from build123d import *

# Parameters (mm, degrees)
SKETCH1_W                                      = 83.2
SKETCH1_H                                      = 74.2
BOSS_EXTRUDE1_DEPTH                            = 8
SHELL1_T                                       = -2
SKETCH2_R                                      = 4.5
SKETCH2_R_2                                    = 2.5
BOSS_EXTRUDE2_DEPTH                            = 4.6
SKETCH3_W                                      = 81.2
SKETCH3_H                                      = 72.2
CUT_EXTRUDE1_DEPTH                             = 1
SKETCH4_R                                      = 2.5
BOSS_EXTRUDE3_DEPTH                            = 0.5
CSK_FOR_M3_FLAT_HEAD_MACHINE_SCREW1_AT_2_COUNT = 2
CSK_FOR_M3_FLAT_HEAD_MACHINE_SCREW1_AT_2_PITCH = 45.11064176
CSK_FOR_M3_FLAT_HEAD_MACHINE_SCREW1_AT_3_COUNT = 2
CSK_FOR_M3_FLAT_HEAD_MACHINE_SCREW1_AT_3_PITCH = 45.11064176
CSK_FOR_M3_FLAT_HEAD_MACHINE_SCREW1_AT_4_COUNT = 2
CSK_FOR_M3_FLAT_HEAD_MACHINE_SCREW1_AT_4_PITCH = 58.2
FILLET1_R                                      = 2


with BuildPart() as part:
    # Sketch1 → Boss-Extrude1 (new body)
    with BuildSketch(Plane(origin=(0, 0, 0), x_dir=(1, 0, 0), z_dir=(0, 1, 0))):
        with Locations((41.6, 37.1)):
            Rectangle(SKETCH1_W, SKETCH1_H)
    extrude(amount=BOSS_EXTRUDE1_DEPTH)

    # Shell1
    shell1_openings = [part.faces().sort_by_distance(p)[0] for p in [
        (41.6, 8, -37.1),
    ]]
    offset(amount=SHELL1_T, openings=shell1_openings, kind=Kind.INTERSECTION)

    # Sketch2 → Boss-Extrude2 (add)
    # profile 1 of 4: a face of its own
    with BuildSketch(Plane(origin=(0, 2, 0), x_dir=(1, 0, 0), z_dir=(0, 1, 0))):
        with Locations(Location((6.6, 67.1, 0), (0, 0, 90))):
            Circle(SKETCH2_R)
        with Locations(Location((6.6, 67.1, 0), (0, 0, 90))):
            Circle(SKETCH2_R_2, mode=Mode.SUBTRACT)
    # profile 2 of 4: a face of its own
    with BuildSketch(Plane(origin=(0, 2, 0), x_dir=(1, 0, 0), z_dir=(0, 1, 0))):
        with Locations(Location((36.6, 26.1, 0), (0, 0, 90))):
            Circle(SKETCH2_R)
        with Locations(Location((36.6, 26.1, 0), (0, 0, 90))):
            Circle(SKETCH2_R_2, mode=Mode.SUBTRACT)
    # profile 3 of 4: a face of its own
    with BuildSketch(Plane(origin=(0, 2, 0), x_dir=(1, 0, 0), z_dir=(0, 1, 0))):
        with Locations((77.6, 67.1)):
            Circle(SKETCH2_R)
        with Locations(Location((77.6, 67.1, 0), (0, 0, 90))):
            Circle(SKETCH2_R_2, mode=Mode.SUBTRACT)
    # profile 4 of 4: a face of its own
    with BuildSketch(Plane(origin=(0, 2, 0), x_dir=(1, 0, 0), z_dir=(0, 1, 0))):
        with Locations((77.6, 21.1)):
            Circle(SKETCH2_R)
        with Locations(Location((77.6, 21.1, 0), (0, 0, 90))):
            Circle(SKETCH2_R_2, mode=Mode.SUBTRACT)
    extrude(amount=BOSS_EXTRUDE2_DEPTH)

    # Sketch3 → Cut-Extrude1 (cut)
    with BuildSketch(Plane(origin=(0, 8, 0), x_dir=(1, 0, 0), z_dir=(0, 1, 0))):
        with Locations((41.6, 37.1)):
            Rectangle(SKETCH3_W, SKETCH3_H)
    extrude(amount=-CUT_EXTRUDE1_DEPTH, mode=Mode.SUBTRACT)

    # Sketch4 → Boss-Extrude3 (add)
    with BuildSketch(Plane(origin=(0, 2, 0), x_dir=(1, 0, 0), z_dir=(0, 1, 0))):
        with Locations(Location((6.6, 67.1, 0), (0, 0, 90))):
            Circle(SKETCH4_R)
        with Locations(Location((77.6, 67.1, 0), (0, 0, 90))):
            Circle(SKETCH4_R)
        with Locations(Location((36.6, 26.1, 0), (0, 0, 90))):
            Circle(SKETCH4_R)
        with Locations(Location((77.6, 21.1, 0), (0, 0, 90))):
            Circle(SKETCH4_R)
    extrude(amount=BOSS_EXTRUDE3_DEPTH)

    # Sketch6 → CSK for M3 Flat Head Machine Screw1 (revolve, cut)
    with BuildSketch(Plane(origin=(41.6, 2, -66.2), x_dir=(0, 0, 1), z_dir=(1, 0, 0))):
        Polygon((0, 0), (0, 2), (1.6, 2), (1.6, 1.55), (3.15, 0), align=None)
    csk_for_m3_flat_head_machine_screw1 = revolve(axis=Axis((41.6, 8.35, -66.2), (0, -1, 0)), mode=Mode.SUBTRACT)

    # CSK for M3 Flat Head Machine Screw1 at 2: CSK for M3 Flat Head Machine Screw1 ×2
    with Locations(*[Vector(-0.7448353357230582, 0, 0.6672483215852396) * (i * CSK_FOR_M3_FLAT_HEAD_MACHINE_SCREW1_AT_2_PITCH) for i in range(1, CSK_FOR_M3_FLAT_HEAD_MACHINE_SCREW1_AT_2_COUNT)]):
        add(csk_for_m3_flat_head_machine_screw1, mode=Mode.SUBTRACT)

    # CSK for M3 Flat Head Machine Screw1 at 3: CSK for M3 Flat Head Machine Screw1 ×2
    with Locations(*[Vector(0.7448353357230579, 0, 0.6672483215852397) * (i * CSK_FOR_M3_FLAT_HEAD_MACHINE_SCREW1_AT_3_PITCH) for i in range(1, CSK_FOR_M3_FLAT_HEAD_MACHINE_SCREW1_AT_3_COUNT)]):
        add(csk_for_m3_flat_head_machine_screw1, mode=Mode.SUBTRACT)

    # CSK for M3 Flat Head Machine Screw1 at 4: CSK for M3 Flat Head Machine Screw1 ×2
    with Locations(*[(0, 0, i * CSK_FOR_M3_FLAT_HEAD_MACHINE_SCREW1_AT_4_PITCH) for i in range(1, CSK_FOR_M3_FLAT_HEAD_MACHINE_SCREW1_AT_4_COUNT)]):
        add(csk_for_m3_flat_head_machine_screw1, mode=Mode.SUBTRACT)

    # Fillet1
    fillet1_edges = [part.edges().sort_by_distance(p)[0] for p in [
        (0, 4, -74.2),
        (83.2, 4, -74.2),
        (83.2, 4, 0),
        (0, 4, 0),
    ]]
    fillet(fillet1_edges, radius=FILLET1_R)


solid = part.part
Input: part model. Units: mm. Frame: model coordinates. A direction names the side the tool comes from. Give positions to 0.01 mm unless a question says otherwise; leave off trailing zeros. Write each loop counter-clockwise with the first axis right and the second up, starting at its lowest first coordinate (ties: lowest second). Pieces come first, ordered by that corner, then holes.
Q1. Section B-B, the plane z = -36.1. Output: boundary loops of the cut face in (x, y), plus the area to 3 significant figures.
Q2. Section D-D, the plane z = -57. Output: boundary loops of the cut face in (x, y), plus the area to 3 significant figures.
Q3. Section A-A, the plane y = 4.75. Output: boundary loops of the cut face in (x, z).
Q4. Section C-C, the plane x = 27. Output: boundary loops of the cut face in (y, z), plus the area to 3 significant figures.
Q5. Pull-direction query (X, two-part tool) for faces 1 (the face through (41, 4, -74.2)), 2 (the face through (0, 4, -37)), 3 (the face through (39, 6.6, -28)); classes: pulls with the +X half, pulls with the -X half, needs draft (parallel to the pull), parting line crosses it, or undercut.
Q6. First-contact query: P1, Ø4.5, axis at x = 38, z = -28, coming from the +Y side; P2, Ø1, axis at x = 67.5, z = -12, coming from the +Y side; P3, Ø1.5, axis at x = 7.5, z = -67.5, coming from the +Y side. Flat tips, straight axial feed; report the tip coordinate or a pass-through.
Q7. Material intervals for probe 1 along Z at (x, y) = (41.6, 0.15); probe 2 along Z at (x, y) = (36.5, 6.25); probe 3 along X at (y, z) = (5.8, -26.1), sorted ascending.
Q8. Set-up query: faces 4 (the face through (75, 6.6, -22)), 5 (the face through (0.57, 4.06, -73.6)). Return all of +Z, -Z, +X, -X, +Y, -Y with unobstructed straight access to the full face (end or side cutting, diameter ignored); none if empty.
Filled in:
1. outline: (0, 0) - (6.4, 0) - (6.4, 0.45) - (4.85, 2) - (2, 2) - (2, 7) - (1, 7) - (1, 8) - (0, 8) - close; (9.6, 0) - (73.6, 0) - (73.6, 0.45) - (72.05, 2) - (11.15, 2) - (9.6, 0.45) - close; (76.8, 0) - (83.2, 0) - (83.2, 8) - (82.2, 8) - (82.2, 7) - (81.2, 7) - (81.2, 2) - (78.35, 2) - (76.8, 0.45) - close
1. area: 171 mm2
2. outline: (0, 0) - (83.2, 0) - (83.2, 8) - (82.2, 8) - (82.2, 7) - (81.2, 7) - (81.2, 2) - (2, 2) - (2, 7) - (1, 7) - (1, 8) - (0, 8) - close
2. area: 188 mm2
3. outline: (0, -72.2) arc R2 ccw to (2, -74.2) - (81.2, -74.2) arc R2 ccw to (83.2, -72.2) - (83.2, -2) arc R2 ccw to (81.2, 0) - (2, 0) arc R2 ccw to (0, -2) - close; circle Ø9 at (6.6, -67.1); circle Ø9 at (36.6, -26.1); hole (2, -72.2) - (81.2, -72.2) - (81.2, -69.8) arc R4.5 cw (long way) to (81.2, -64.4) - (81.2, -23.8) arc R4.5 cw (long way) to (81.2, -18.4) - (81.2, -2) - (2, -2) - close; hole circle Ø5 at (6.6, -67.1); hole circle Ø5 at (36.6, -26.1); hole circle Ø5 at (77.6, -67.1); hole circle Ø5 at (77.6, -21.1)
4. outline: (0, -74.2) - (8, -74.2) - (8, -73.2) - (7, -73.2) - (7, -72.2) - (2, -72.2) - (2, -2) - (7, -2) - (7, -1) - (8, -1) - (8, 0) - (0, 0) - close
4. area: 170 mm2
5. face 1: needs draft
5. face 2: pulls with the -X half
5. face 3: undercut
6. P1: stops at y = 6.6
6. P2: stops at y = 2
6. P3: stops at y = 2.5
7. probe 1: z = -74.2 to -67.8, -64.6 to -9.6, -6.4 to 0
7. probe 2: z = -74.2 to -72.2, -30.6 to -28.6, -23.6 to -21.6, -2 to 0
7. probe 3: x = 0 to 2, 32.1 to 34.1, 39.1 to 41.1, 81.2 to 83.2
8. face 4: +Y
8. face 5: -Z, -X, +Y, -Y
